Build history of the part. All positions in model axes, mm. A direction names the side the tool comes from. Coordinates: 2 decimals unless noted, no trailing zeros. Loops run counter-clockwise (first coordinate to the right, second up) from the corner with the lowest first, then second, coordinate; pieces in that order, holes last.
(1) Flat gauge pin, fed straight in: P1, Ø2, axis at x = -75.5, z = 91, coming from the +Y side. Where does the tip first touch, or does it go through?
(2) Two-plate mould, pull along Z, no slides. Class faces 4 (the face through (-75, 28, 97)), 5 (the face through (-75, 15, 124.893)), 6 (the face through (-76.669, 15, 46)), 7 (the face through (-75, 2, 12.674)): pulls with the +Z half, pulls with the -Z half, needs draft (parallel to the pull), parting line crosses it, or undercut.
(3) Slice it at C-C (z = 79). Give the cut face in (x, y).
(4) Slice it at A-A (y = 27.75). Give the cut face in (x, z).
(5) Tool access for faces 1 (the face through (-75, 26, 80)), 2 (the face through (-75, 4, -4)), 3 (the face through (-75, 30, 22)): list every direction of +Z, -Z, +X, -X, +Y, -Y with a clear straight run to the whole face (end or side of a thin tool).
(6) Wall check: L1, parallel to Z at x = -74.7, y = 2; L2, parallel to Z at x = -73.85, y = 28.25; L3, parallel to Y at x = -76.1, z = -1. Give the ranges that are in metal, low to high.
(7) Slice it at B-B (x = -73.7). Give the cut face in (y, z), and give its area (3 significant figures).
Autodesk Fusion 360 part; units mm, degrees
sketch "Boceto1" plane through (0, 0, 0) normal (0, 1, 0) x (1, 0, 0)
  line L0 (-76.6693, 30.4647) -> (-76.6693, -124.8933)
  line L1 (-95, 0) -> (105, 0) construction
  line L2 (-76.6693, 30.4647) -> (-72.6693, 30.4647)
  line L3 (-72.6693, 30.4647) -> (-72.6693, -124.8933)
  line L4 (-76.6693, -124.8933) -> (-72.6693, -124.8933)
  dimension "d59" = 4
extrude "Extruir1" add sketch "Boceto1" along normal blind 30
sketch "Boceto2" plane through (-72.6693, 0, 0) normal (1, 0, 0) x (0, 0, -1)
  line L0 (-124.8933, 0) -> (30.4647, 0)
  line L1 (30.4647, 0) -> (30.4647, 30)
  line L2 (30.4647, 30) -> (-124.8933, 30)
  line L3 (-124.8933, 30) -> (-124.8933, 0)
  line L4 (-76, 30) -> (-84, 30)
  line L5 (-84, 26) -> (-76, 26)
  line L6 (-76, 26) -> (-76, 30)
  line L7 (-89, 30) -> (-97, 30)
  line L8 (-97, 30) -> (-97, 28)
  line L9 (-89, 28) -> (-89, 30)
  line L10 (-97, 26) -> (-89, 26)
  line L11 (-89, 26) -> (-89, 30)
  line L12 (-76, 30) -> (-84, 30)
  line L13 (-97, 30) -> (-97, 26)
  line L14 (8.3256, 0) -> (0.3256, 0)
  line L15 (0.3256, 0) -> (0.3256, 4)
  line L16 (0.3256, 4) -> (8.3256, 4)
  line L17 (8.3256, 4) -> (8.3256, 0)
  line L18 (-4.6744, 0) -> (-12.6744, 0)
  line L19 (-12.6744, 0) -> (-12.6744, 4)
  line L20 (-12.6744, 4) -> (-4.6744, 4)
  line L21 (-4.6744, 4) -> (-4.6744, 0)
  line L22 (-84, 30) -> (-84, 26)
  dimension "d43" = 8
  dimension "d46" = 8
  dimension "d47" = 4
  dimension "d50" = 4
  dimension "d51" = 8
  dimension "d52" = 5
  dimension "d53" = 4
  dimension "d54" = 5
  dimension "d55" = 8
  dimension "d56" = 8
  dimension "d57" = 4
extrude "Extruir2" cut sketch "Boceto2" against normal through all contours L0 L18 L19 L20 L21 | L2 L7 L8 L9 L10 L11 L13 | L0 L14 L15 L16 L17 | L2 L4 L5 L6 L12 L22
sketch "Boceto3" plane through (-72.6693, 0, 0) normal (1, 0, 0) x (0, 0, -1)
  line L0 (-12.6744, 0) -> (-12.6744, 4)
  line L1 (-12.6744, 4) -> (-4.6744, 4)
  line L2 (-4.6744, 4) -> (-4.6744, 0)
  line L3 (-4.6744, 0) -> (0.3256, 0)
  line L4 (0.3256, 0) -> (0.3256, 4)
  line L5 (0.3256, 4) -> (8.3256, 4)
  line L6 (8.3256, 4) -> (8.3256, 0)
  line L7 (8.3256, 0) -> (30.4647, 0)
  line L8 (30.4647, 0) -> (30.4647, 30)
  line L9 (30.4647, 30) -> (-76, 30)
  line L10 (-76, 30) -> (-76, 26)
  line L11 (-76, 26) -> (-84, 26)
  line L12 (-84, 26) -> (-84, 30)
  line L13 (-84, 30) -> (-89, 30)
  line L14 (-89, 30) -> (-89, 26)
  line L15 (-89, 26) -> (-97, 26)
  line L16 (-97, 26) -> (-97, 30)
  line L17 (-97, 30) -> (-124.8933, 30)
  line L18 (-124.8933, 30) -> (-124.8933, 0)
  line L19 (-124.8933, 0) -> (-12.6744, 0)
  line L20 (-4.6744, 0) -> (-4.6744, 4)
  line L21 (-4.6744, 4) -> (-12.6744, 4)
  line L22 (-12.6744, 4) -> (-12.6744, 0)
  line L23 (-97, 30) -> (-97, 26)
  line L24 (-97, 26) -> (-89, 26)
  line L25 (-89, 26) -> (-89, 30)
  line L26 (8.3256, 0) -> (8.3256, 4)
  line L27 (8.3256, 4) -> (0.3256, 4)
  line L28 (0.3256, 4) -> (0.3256, 0)
  line L29 (-84, 30) -> (-84, 26)
  line L30 (-84, 26) -> (-76, 26)
  line L31 (-76, 26) -> (-76, 30)
  line L32 (30.4647, 0) -> (8.3256, 0)
  line L33 (0.3256, 0) -> (-4.6744, 0)
  line L34 (-97, 30) -> (-124.8933, 30)
  line L35 (30.4647, 30) -> (-76, 30)
  line L36 (30.4647, 0) -> (30.4647, 30)
  line L37 (-124.8933, 0) -> (-124.8933, 30)
  line L38 (-12.6744, 0) -> (-124.8933, 0)
  line L39 (-84, 30) -> (-89, 30)
Response values:
1. P1: stops at y = 26
2. face 4: undercut
2. face 5: pulls with the +Z half
2. face 6: needs draft
2. face 7: undercut
3. outline: (-76.67, 0) - (-72.67, 0) - (-72.67, 26) - (-76.67, 26) - close
4. outline: (-76.67, -30.46) - (-72.67, -30.46) - (-72.67, 76) - (-76.67, 76) - close; (-76.67, 84) - (-72.67, 84) - (-72.67, 89) - (-76.67, 89) - close; (-76.67, 97) - (-72.67, 97) - (-72.67, 124.89) - (-76.67, 124.89) - close
5. face 1: +X, -X, +Y
5. face 2: +X, -X, -Y
5. face 3: +Z, -Z, +X, -X, +Y
6. L1: z = -30.46 to -8.33, -0.33 to 4.67, 12.67 to 124.89
6. L2: z = -30.46 to 76, 84 to 89, 97 to 124.89
6. L3: y = 4 to 30
7. outline: (0, -30.46) - (30, -30.46) - (30, 76) - (26, 76) - (26, 84) - (30, 84) - (30, 89) - (26, 89) - (26, 97) - (30, 97) - (30, 124.89) - (0, 124.89) - (0, 12.67) - (4, 12.67) - (4, 4.67) - (0, 4.67) - (0, -0.33) - (4, -0.33) - (4, -8.33) - (0, -8.33) - close
7. area: 4,530 mm2
